Can you work these out from the model? Positions are in its coordinate system, mm. Face numbers are marked on the shaded views. Give positions to 0.01 mm unless a question says otherwise; leave off trailing zeros.
from build123d import *

# Parameters (mm, degrees)
SKETCH1_R           = 5
BOSS_EXTRUDE2_DEPTH = 1
BOSS_EXTRUDE3_DEPTH = 5
BOSS_EXTRUDE4_DEPTH = 3
FILLET1_SIZE        = 5
FILLET1_SIZE_2      = 3
FILLET2_SIZE        = 5
FILLET2_SIZE_2      = 3


with BuildPart() as part:
    # Sketch1 → Boss-Extrude2 (new body)
    with BuildSketch(Plane(origin=(0, 0, 0), x_dir=(1, 0, 0), z_dir=(0, 1, 0))):
        with BuildLine():
            ThreePointArc((10, 0), (2.928932188, 2.928932188), (0, 10))
            Line((0, 10), (0, 30))
            ThreePointArc((0, 30), (2.928932188, 37.071067812), (10, 40))
            Line((10, 40), (30, 40))
            ThreePointArc((30, 40), (37.071067812, 37.071067812), (40, 30))
            Line((40, 30), (40, 10))
            ThreePointArc((40, 10), (37.071067812, 2.928932188), (30, 0))
            Line((30, 0), (10, 0))
        make_face()
        with Locations(Location((20, 20, 0), (0, 0, 270))):
            Circle(SKETCH1_R, mode=Mode.SUBTRACT)
    extrude(amount=BOSS_EXTRUDE2_DEPTH)

    # Sketch1<4> → Boss-Extrude3 (add)
    with BuildSketch(Plane(origin=(0, 0, 0), x_dir=(1, 0, 0), z_dir=(0, 1, 0))):
        with BuildLine():
            ThreePointArc((10, -1), (2.221825407, 2.221825407), (-1, 10))
            Line((-1, 10), (-1, 30))
            ThreePointArc((-1, 30), (2.221825407, 37.778174593), (10, 41))
            Line((10, 41), (30, 41))
            ThreePointArc((30, 41), (37.778174593, 37.778174593), (41, 30))
            Line((41, 30), (41, 10))
            ThreePointArc((41, 10), (37.778174593, 2.221825407), (30, -1))
            Line((30, -1), (10, -1))
        make_face()
        with BuildLine():
            Line((10, 0), (30, 0))
            ThreePointArc((30, 0), (37.071067812, 2.928932188), (40, 10))
            Line((40, 10), (40, 30))
            ThreePointArc((40, 30), (37.071067812, 37.071067812), (30, 40))
            Line((30, 40), (10, 40))
            ThreePointArc((10, 40), (2.928932188, 37.071067812), (0, 30))
            Line((0, 30), (0, 10))
            ThreePointArc((0, 10), (2.928932188, 2.928932188), (10, 0))
        make_face(mode=Mode.SUBTRACT)
    extrude(amount=BOSS_EXTRUDE3_DEPTH)

    # Sketch1<5> → Boss-Extrude4 (add)
    with BuildSketch(Plane(origin=(0, 0, 0), x_dir=(1, 0, 0), z_dir=(0, 1, 0))):
        with BuildLine():
            ThreePointArc((10, -2), (1.514718626, 1.514718626), (-2, 10))
            Line((-2, 10), (-2, 30))
            ThreePointArc((-2, 30), (1.514718626, 38.485281374), (10, 42))
            Line((10, 42), (30, 42))
            ThreePointArc((30, 42), (38.485281374, 38.485281374), (42, 30))
            Line((42, 30), (42, 10))
            ThreePointArc((42, 10), (38.485281374, 1.514718626), (30, -2))
            Line((30, -2), (10, -2))
        make_face()
        with BuildLine():
            Line((10, -1), (30, -1))
            ThreePointArc((30, -1), (37.778174593, 2.221825407), (41, 10))
            Line((41, 10), (41, 30))
            ThreePointArc((41, 30), (37.778174593, 37.778174593), (30, 41))
            Line((30, 41), (10, 41))
            ThreePointArc((10, 41), (2.221825407, 37.778174593), (-1, 30))
            Line((-1, 30), (-1, 10))
            ThreePointArc((-1, 10), (2.221825407, 2.221825407), (10, -1))
        make_face(mode=Mode.SUBTRACT)
    extrude(amount=BOSS_EXTRUDE4_DEPTH)

    # Fillet1
    # an asymmetric fillet: 5, 3 mm, written as the material it adds along each edge
    with BuildSketch(Plane(origin=(10, 1, -10), x_dir=(0, 0, 1), z_dir=(1, 0, 0))) as fillet1_piece_1:
        with BuildLine():
            Bezier((10 - FILLET1_SIZE, 0), (10, 0), (10, -FILLET1_SIZE_2), weights=[1, 0.707106781, 1])
            Line((10, -FILLET1_SIZE_2), (10, 0))
            Line((10, 0), (10 - FILLET1_SIZE, 0))
        make_face()
    revolve(axis=Axis((10, 1, -10), (0, -1, 0)), revolution_arc=90)
    with BuildSketch(Plane(origin=(30, 1, 0), x_dir=(0, 0, -1), z_dir=(-1, 0, 0)), Plane(origin=(40, 1, -30), x_dir=(-1, 0, 0), z_dir=(0, 0, 1)), Plane(origin=(10, 1, -40), x_dir=(0, 0, 1), z_dir=(1, 0, 0)), Plane(origin=(0, 1, -10), x_dir=(1, 0, 0), z_dir=(0, 0, -1))) as fillet1_piece_2:
        with BuildLine():
            Bezier((FILLET1_SIZE, 0), (0, 0), (0, -FILLET1_SIZE_2), weights=[1, 0.707106781, 1])
            Line((0, -FILLET1_SIZE_2), (0, 0))
            Line((0, 0), (FILLET1_SIZE, 0))
        make_face()
    extrude(amount=20)
    with BuildSketch(Plane(origin=(30, 1, -10), x_dir=(1, 0, 0), z_dir=(0, 0, -1))) as fillet1_piece_3:
        with BuildLine():
            Bezier((10 - FILLET1_SIZE, 0), (10, 0), (10, -FILLET1_SIZE_2), weights=[1, 0.707106781, 1])
            Line((10, -FILLET1_SIZE_2), (10, 0))
            Line((10, 0), (10 - FILLET1_SIZE, 0))
        make_face()
    revolve(axis=Axis((30, 1, -10), (0, -1, 0)), revolution_arc=90)
    with BuildSketch(Plane(origin=(30, 1, -30), x_dir=(0, 0, -1), z_dir=(-1, 0, 0))) as fillet1_piece_4:
        with BuildLine():
            Bezier((10 - FILLET1_SIZE, 0), (10, 0), (10, -FILLET1_SIZE_2), weights=[1, 0.707106781, 1])
            Line((10, -FILLET1_SIZE_2), (10, 0))
            Line((10, 0), (10 - FILLET1_SIZE, 0))
        make_face()
    revolve(axis=Axis((30, 1, -30), (0, -1, 0)), revolution_arc=90)
    with BuildSketch(Plane(origin=(10, 1, -30), x_dir=(-1, 0, 0), z_dir=(0, 0, 1))) as fillet1_piece_5:
        with BuildLine():
            Bezier((10 - FILLET1_SIZE, 0), (10, 0), (10, -FILLET1_SIZE_2), weights=[1, 0.707106781, 1])
            Line((10, -FILLET1_SIZE_2), (10, 0))
            Line((10, 0), (10 - FILLET1_SIZE, 0))
        make_face()
    revolve(axis=Axis((10, 1, -30), (0, -1, 0)), revolution_arc=90)

    # Fillet2
    # an asymmetric fillet: 5, 3 mm, written as the material it takes off along each edge
    with BuildSketch(Plane(origin=(10, 0, -42), x_dir=(0, 0, 1), z_dir=(1, 0, 0)), Plane(origin=(-2, 0, -10), x_dir=(1, 0, 0), z_dir=(0, 0, -1)), Plane(origin=(42, 0, -30), x_dir=(-1, 0, 0), z_dir=(0, 0, 1)), Plane(origin=(30, 0, 2), x_dir=(0, 0, -1), z_dir=(-1, 0, 0))) as fillet2_piece_1:
        with BuildLine():
            Bezier((FILLET2_SIZE, 0), (0, 0), (0, -FILLET2_SIZE_2), weights=[1, 0.707106781, 1])
            Line((0, -FILLET2_SIZE_2), (-0.1, -3))
            Line((-0.1, -3), (-0.1, 0.1))
            Line((-0.1, 0.1), (5, 0.1))
            Line((5, 0.1), (FILLET2_SIZE, 0))
        make_face()
    extrude(amount=20, mode=Mode.SUBTRACT)
    with BuildSketch(Plane(origin=(10, 0, -30), x_dir=(-1, 0, 0), z_dir=(0, 0, 1))) as fillet2_piece_2:
        with BuildLine():
            Bezier((12 - FILLET2_SIZE, 0), (12, 0), (12, -FILLET2_SIZE_2), weights=[1, 0.707106781, 1])
            Line((12, -FILLET2_SIZE_2), (12.1, -3))
            Line((12.1, -3), (12.1, 0.1))
            Line((12.1, 0.1), (7, 0.1))
            Line((7, 0.1), (12 - FILLET2_SIZE, 0))
        make_face()
    revolve(axis=Axis((10, 0, -30), (0, -1, 0)), revolution_arc=90, mode=Mode.SUBTRACT)
    with BuildSketch(Plane(origin=(30, 0, -30), x_dir=(0, 0, -1), z_dir=(-1, 0, 0))) as fillet2_piece_3:
        with BuildLine():
            Bezier((12 - FILLET2_SIZE, 0), (12, 0), (12, -FILLET2_SIZE_2), weights=[1, 0.707106781, 1])
            Line((12, -FILLET2_SIZE_2), (12.1, -3))
            Line((12.1, -3), (12.1, 0.1))
            Line((12.1, 0.1), (7, 0.1))
            Line((7, 0.1), (12 - FILLET2_SIZE, 0))
        make_face()
    revolve(axis=Axis((30, 0, -30), (0, -1, 0)), revolution_arc=90, mode=Mode.SUBTRACT)
    with BuildSketch(Plane(origin=(10, 0, -10), x_dir=(0, 0, 1), z_dir=(1, 0, 0))) as fillet2_piece_4:
        with BuildLine():
            Bezier((12 - FILLET2_SIZE, 0), (12, 0), (12, -FILLET2_SIZE_2), weights=[1, 0.707106781, 1])
            Line((12, -FILLET2_SIZE_2), (12.1, -3))
            Line((12.1, -3), (12.1, 0.1))
            Line((12.1, 0.1), (7, 0.1))
            Line((7, 0.1), (12 - FILLET2_SIZE, 0))
        make_face()
    revolve(axis=Axis((10, 0, -10), (0, -1, 0)), revolution_arc=90, mode=Mode.SUBTRACT)
    with BuildSketch(Plane(origin=(30, 0, -10), x_dir=(1, 0, 0), z_dir=(0, 0, -1))) as fillet2_piece_5:
        with BuildLine():
            Bezier((12 - FILLET2_SIZE, 0), (12, 0), (12, -FILLET2_SIZE_2), weights=[1, 0.707106781, 1])
            Line((12, -FILLET2_SIZE_2), (12.1, -3))
            Line((12.1, -3), (12.1, 0.1))
            Line((12.1, 0.1), (7, 0.1))
            Line((7, 0.1), (12 - FILLET2_SIZE, 0))
        make_face()
    revolve(axis=Axis((30, 0, -10), (0, -1, 0)), revolution_arc=90, mode=Mode.SUBTRACT)


solid = part.part
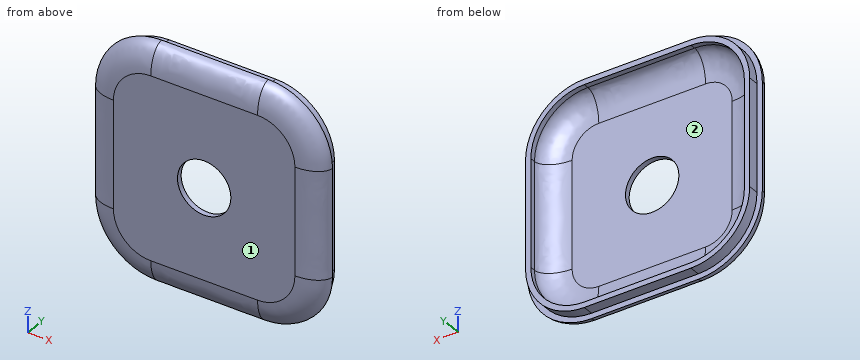
(1) If I drill on L1, parallel to X at y = 4.3, z = -23; L2, parallel to Z at x = 31, y = 1.7; L3, parallel to Y at x = 14, z = -31.5, over which ranges is the centre line in solid material (lowest first)?
Returned:
L1: x = -1 to 0, 40 to 41
L2: z = -41.46 to -38.15, -1.85 to 1.46
L3: y = 0 to 1
(2) Will these pins go through, and if not, where does the flat tip stop? P1, Ø4, axis at x = 11.5, z = -29, coming from the +Y side; P2, Ø22, axis at x = 16.5, z = -25.5, coming from the +Y side; P3, Ø2, axis at x = 36.5, y = 2.5, coming from the -Z side; P4, Ø8, axis at x = 20, z = -20, coming from the -Y side.
Returned:
P1: stops at y = 1
P2: stops at y = 1.14
P3: stops at z = -40.63
P4: passes through
(3) If we mould it in two halves opening along Z, with no side actions, what happens to the marked faces 1 and 2? For each: +Z half, -Z half, draft (parallel to the pull), parting line (faces both ways), or undercut.
Returned:
face 1: draft
face 2: undercut
